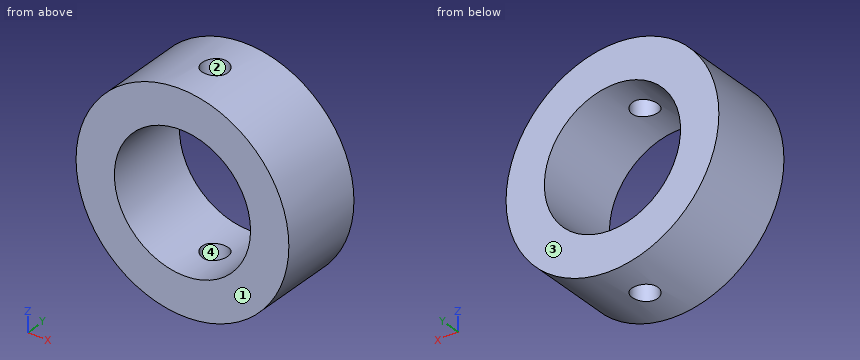
```python
from build123d import *

# Parameters (mm, degrees)
SKETCH2_R               = 12.5
BOSS_EXTRUDE1_DEPTH     = 10
SKETCH3_R               = 8
CUT_EXTRUDE1_DEPTH      = 10
SKETCH5_R               = 1.5
CUT_EXTRUDE2_DEPTH      = 13.5
CUT_EXTRUDE2_DEPTH_BACK = 13.5
SCALE1_SCALE            = 2


with BuildPart() as part:
    # Sketch2 → Boss-Extrude1 (new body)
    with BuildSketch(Plane(origin=(0, 0, 0), x_dir=(1, 0, 0), z_dir=(0, 1, 0))):
        Circle(SKETCH2_R)
    extrude(amount=BOSS_EXTRUDE1_DEPTH)

    # Sketch3 → Cut-Extrude1 (cut)
    with BuildSketch(Plane(origin=(0, 10, 0), x_dir=(1, 0, 0), z_dir=(0, 1, 0))):
        Circle(SKETCH3_R)
    extrude(amount=-CUT_EXTRUDE1_DEPTH, mode=Mode.SUBTRACT)

    # Sketch5 → Cut-Extrude2 (cut, two sides)
    with BuildSketch(Plane.XY) as cut_extrude2_sk:
        with Locations((0, 5)):
            Circle(SKETCH5_R)
    extrude(amount=CUT_EXTRUDE2_DEPTH, mode=Mode.SUBTRACT)
    extrude(cut_extrude2_sk.sketch, amount=-CUT_EXTRUDE2_DEPTH_BACK, mode=Mode.SUBTRACT)


with BuildPart() as part_1:
    # Scale1: scaled about (1.973e-06, 5.000003293, 0)
    add(part.part.scale(SCALE1_SCALE).moved(Location((-1.973e-06, -5.000003293, 0))))


solid = part_1.part
```
Can you work these out from the model? Positions are in its coordinate system, mm. Face numbers are marked on the shaded views. Give positions to 0.01 mm unless a question says otherwise; leave off trailing zeros. Order: outer loops, then holes, each group sorted by start corner. A loop starts at its lowest first (then second) coordinate and runs counter-clockwise, first axis right, second up. Notation, with made-up numbers: (13.5, 77) - (22.5, 77) arc R24 cw to (22.5, 104) - close; hole circle Ø6 at (61.5, 72.5). An arc over 180 degrees is marked (long way). Use a Markdown table: item, result. Add a question column.
Q1. I'm going to push flat-ended pins straight in: pin 1 (5 mm diameter, centred on y = -0.5, z = 18, fed in from -X); pin 2 (1.5 mm diameter, centred on x = -2.5, y = 7.5, fed in from +Z); pin 3 (9.5 mm diameter, centred on x = 0, y = 5, fed in from +Z); pin 4 (5 mm diameter, centred on x = 16, y = -0.5, fed in from -Z). Where does each tip first touch, or does it pass through?
Q2. If we section it at D-D on z = 19.5: Write out the boundary of the cut face in (x, y).
Q3. If we section it at B-B on x = 13: Write out the boundary of the cut face in (y, z).
Q4. Please list where these lines run through material, in increasing order: line 1 along X through (y, z) = (0, 0); line 2 along Z through (x, y) = (0.5, 0.25) (3 decimals); line 3 along X through (y, z) = (6.75, -2).
Q5. If we mould it in two halves opening along Y, with no side actions, what happens to the marked faces 1, 2, 3 and 4? For each: released by +Y, released by -Y, zero draft, split by the parting line, or undercut.
Q6. If we section it at C-C on y = -2: Write out the boundary of the cut face in (x, z), plus the area to 3 significant figures.
Q7. If we section it at A-A on z = 0: Write out the boundary of the cut face in (x, y).
Answers follow:
| question | item | result |
|---|---|---|
| 1 | pin 1 | stops at x = -19.62 |
| 1 | pin 2 | stops at z = 24.94 |
| 1 | pin 3 | stops at z = 25 |
| 1 | pin 4 | stops at z = -21.04 |
| 2 | outline | (-15.64, -5) - (15.64, -5) - (15.64, 15) - (-15.64, 15) - close; hole circle Ø6 at (0, 5) |
| 3 | outline | (-5, -21.35) - (15, -21.35) - (15, -9.33) - (-5, -9.33) - close; (-5, 9.33) - (15, 9.33) - (15, 21.35) - (-5, 21.35) - close |
| 4 | line 1 | x = -25 to -16, 16 to 25 |
| 4 | line 2 | z = -24.995 to -15.992, 15.992 to 24.995 |
| 4 | line 3 | x = -24.92 to -15.87, 15.87 to 24.92 |
| 5 | face 1 | released by -Y |
| 5 | face 2 | undercut |
| 5 | face 3 | released by +Y |
| 5 | face 4 | undercut |
| 6 | outline | circle Ø50 at (0, 0); hole circle Ø32 at (0, 0) |
| 6 | area | 1,160 mm^2 |
| 7 | outline | (-25, -5) - (-16, -5) - (-16, 15) - (-25, 15) - close; (16, -5) - (25, -5) - (25, 15) - (16, 15) - close |
